Design review of the part built by this model. Coordinates are the model's own, in mm. A direction names the side the tool comes from. Coordinates: 2 decimals unless noted, no trailing zeros. Write each loop counter-clockwise with the first axis right and the second up, starting at its lowest first coordinate (ties: lowest second). Pieces come first, ordered by that corner, then holes. Notation, with made-up numbers: (40, 83) -> (85, 83) arc R22 cw to (85, 118) -> close; hole circle Ø7 at (2.5, 83.25). An arc over 180 degrees is marked (long way). Answer in a Markdown table with one row per item. Add a question column.
Item 1: Take a section at D-D, the plane x = 65. Write out the cut boundary in (y, z).
Item 2: To check wall thickness, follow line 1 (Z direction, x = -124, y = 12.75); line 2 (Z direction, x = -187, y = 11); line 3 (X direction, y = 25.75, z = 16). State the ranges of each line that lie inside material, in increasing order.
Item 3: Clearance check with flat-ended pins moving along their axes: P1, Ø9, axis at x = -237, z = 0, coming from the +Y side; P2, Ø6, axis at x = -19, z = -0.5, coming from the -Y side; P3, Ø6, axis at x = -152, y = 12.5, coming from the -Z side; P4, Ø4, axis at y = 5.5, z = 5, coming from the +X side. State where each tip first meets the part, or that it passes through.
Item 4: Take a section at C-C, the plane z = 29. Write out the cut boundary in (x, y).
Item 5: Take a section at A-A, the plane x = -77. Write out the cut boundary in (y, z), and give its area (3 significant figures).
Item 6: For faces 1 (the face through (80.096, 20.14, -5.42)), 2 (the face through (-234, 21, 0)), 3 (the face through (-98, 15, -17.5)), list the 3-axis set-ups (+Z, -Z, +X, -X, +Y, -Y) from which the entire face can be reached by the end or side of a thin tool; tool diameter is ignored.
Item 7: Draft analysis for pull direction X (two halves, no side actions). For faces 4 (the face through (144.484, 15.21, 1.174)), 5 (the face through (-124, 15, -9.538)), 6 (the face through (-98, 15, 17.5)), state which applies: released by +X, released by -X, zero draft, split by the parting line, or undercut.
Item 8: Take a section at B-B, the plane y = 26.5. Write out the cut boundary in (x, z).
from build123d import *

# Parameters (mm, degrees)
SKETCH2_W           = 247
SKETCH2_H           = 35
BOSS_EXTRUDE1_DEPTH = 30
SKETCH3_R           = 5.6
CUT_EXTRUDE1_DEPTH  = 250.429849858
CUT_EXTRUDE2_DEPTH  = 22
SKETCH6_W           = 22.496439662
SKETCH6_H           = 14
BOSS_EXTRUDE3_DEPTH = 38
CUT_EXTRUDE4_DEPTH  = 17.5
SKETCH9_R           = 2
CUT_EXTRUDE5_DEPTH  = 38
SKETCH15_R          = 2.75
CUT_EXTRUDE10_DEPTH = 9
CUT_EXTRUDE11_DEPTH = 21
SKETCH17_W          = 129.66543269
SKETCH17_H          = 19.076880406
CUT_EXTRUDE12_DEPTH = 250.429849858
FILLET1_R           = 10
SKETCH19_W          = 35
SKETCH19_H          = 30
BOSS_EXTRUDE5_DEPTH = 55
BOSS_EXTRUDE4_DEPTH = 30
SKETCH21_R          = 25
CUT_EXTRUDE14_DEPTH = 20


with BuildPart() as part:
    # Sketch2 → Boss-Extrude1 (new body)
    with BuildSketch(Plane(origin=(0, 0, 0), x_dir=(1, 0, 0), z_dir=(0, 1, 0))):
        with Locations((-123.5, 0)):
            Rectangle(SKETCH2_W, SKETCH2_H)
    extrude(amount=BOSS_EXTRUDE1_DEPTH)

    # Sketch3 → Cut-Extrude1 (cut, through all)
    with BuildSketch(Plane.XZ):
        with Locations(Location((-21, 0, 0), (0, 0, 270))):
            Circle(SKETCH3_R)
    extrude(amount=-CUT_EXTRUDE1_DEPTH, mode=Mode.SUBTRACT)

    # Sketch4 → Cut-Extrude2 (cut)
    with BuildSketch(Plane(origin=(0, 30, 0), x_dir=(1, 0, 0), z_dir=(0, 1, 0))):
        Polygon((-14.9, 3.521836642), (-21, 7.043673284), (-27.1, 3.521836642), (-27.1, -3.521836642), (-21, -7.043673284), (-14.9, -3.521836642), align=None)
    extrude(amount=-CUT_EXTRUDE2_DEPTH, mode=Mode.SUBTRACT)

    # Sketch6 → Boss-Extrude3 (add)
    with BuildSketch(Plane(origin=(0, 0, 0), x_dir=(0, 0, -1), z_dir=(1, 0, 0))):
        with Locations((0.204742288, 23)):
            Rectangle(SKETCH6_W, SKETCH6_H)
    extrude(amount=-BOSS_EXTRUDE3_DEPTH)

    # Sketch7 → Cut-Extrude4 (cut)
    with BuildSketch(Plane.XY.offset(17.5)):
        Polygon((-21, 16), (-14.9, 16), (-14.9, 8), (-15.4, 8), (-15.4, 0), (-26.6, 0), (-26.6, 8), (-27.1, 8), (-27.1, 16), align=None)
    extrude(amount=-CUT_EXTRUDE4_DEPTH, mode=Mode.SUBTRACT)

    # Sketch9 → Cut-Extrude5 (cut)
    with BuildSketch(Plane(origin=(0, 30, 0), x_dir=(1, 0, 0), z_dir=(0, 1, 0))):
        with Locations(Location((-21, 0, 0), (0, 0, 270))):
            Circle(SKETCH9_R)
    extrude(amount=-CUT_EXTRUDE5_DEPTH, mode=Mode.SUBTRACT)

    # Sketch15 → Cut-Extrude10 (cut)
    with BuildSketch(Plane(origin=(0, 30, 0), x_dir=(1, 0, 0), z_dir=(0, 1, 0))):
        with Locations(Location((-237, 0, 0), (0, 0, 270))):
            Circle(SKETCH15_R)
    extrude(amount=-CUT_EXTRUDE10_DEPTH, mode=Mode.SUBTRACT)

    # Sketch16 → Cut-Extrude11 (cut)
    with BuildSketch(Plane.XZ):
        Polygon((-241.130206964, 2.650419546), (-241.36043414, -2.25165438), (-237.230227176, -4.902073926), (-232.869793036, -2.650419546), (-232.63956586, 2.25165438), (-236.769772824, 4.902073926), align=None)
    extrude(amount=-CUT_EXTRUDE11_DEPTH, mode=Mode.SUBTRACT)

    # Sketch17 → Cut-Extrude12 (cut, through all)
    with BuildSketch(Plane(origin=(0, 30, 0), x_dir=(1, 0, 0), z_dir=(0, 1, 0))):
        with Locations((-123.5, 0)):
            Rectangle(SKETCH17_W, SKETCH17_H)
    extrude(amount=-CUT_EXTRUDE12_DEPTH, mode=Mode.SUBTRACT)

    # Fillet1
    # the kernel refuses this fillet: 10 mm, written as the material it adds along each edge
    with BuildSketch(Plane(origin=(-58.667283655, 30, 9.538440203), x_dir=(0, 0, -1), z_dir=(0, -1, 0))) as fillet1_piece_1:
        with BuildLine():
            CenterArc((FILLET1_R, -FILLET1_R), FILLET1_R, 90, 90)
            Line((0, -FILLET1_R), (0, 0))
            Line((0, 0), (FILLET1_R, 0))
        make_face()
    extrude(amount=30)
    with BuildSketch(Plane(origin=(-58.667283655, 30, -9.538440203), x_dir=(0, 0, 1), z_dir=(0, -1, 0)), Plane(origin=(-188.332716345, 30, -9.538440203), x_dir=(1, 0, 0), z_dir=(0, -1, 0)), Plane(origin=(-188.332716345, 30, 9.538440203), x_dir=(0, 0, -1), z_dir=(0, -1, 0))) as fillet1_piece_2:
        with BuildLine():
            CenterArc((FILLET1_R, FILLET1_R), FILLET1_R, 180, 90)
            Line((0, FILLET1_R), (0, 0))
            Line((0, 0), (FILLET1_R, 0))
        make_face()
    extrude(amount=30)

    # Sketch19 → Boss-Extrude5 (add)
    with BuildSketch(Plane(origin=(0, 0, 0), x_dir=(0, 0, -1), z_dir=(1, 0, 0))):
        with Locations((0, 15)):
            Rectangle(SKETCH19_W, SKETCH19_H)
    extrude(amount=BOSS_EXTRUDE5_DEPTH)

    # Sketch18 → Boss-Extrude4 (add)
    with BuildSketch(Plane(origin=(0, 30, 0), x_dir=(1, 0, 0), z_dir=(0, 1, 0))):
        with BuildLine():
            Line((55, 17.5), (55, -17.5))
            Line((55, -17.5), (84.405509337, -34.58567742))
            ThreePointArc((84.405509337, -34.58567742), (144.501054052, 0), (84.405509337, 34.58567742))
            Line((84.405509337, 34.58567742), (55, 17.5))
        make_face()
    extrude(amount=-BOSS_EXTRUDE4_DEPTH)

    # Sketch21 → Cut-Extrude14 (cut)
    with BuildSketch(Plane(origin=(0, 30, 0), x_dir=(1, 0, 0), z_dir=(0, 1, 0))):
        with Locations(Location((104.501054052, 0, 0), (0, 0, 270))):
            Circle(SKETCH21_R)
    extrude(amount=-CUT_EXTRUDE14_DEPTH, mode=Mode.SUBTRACT)


solid = part.part
Answers:
| question | item | result |
|---|---|---|
| 1 | outline | (0, -23.31) -> (30, -23.31) -> (30, 23.31) -> (0, 23.31) -> close |
| 2 | line 1 | z = -17.5 to -9.54, 9.54 to 17.5 |
| 2 | line 2 | z = -17.5 to -4.53, 4.53 to 17.5 |
| 2 | line 3 | x = -247 to 85.29, 123.71 to 141.16 |
| 3 | P1 | stops at y = 30 |
| 3 | P2 | stops at y = 16 |
| 3 | P3 | stops at z = -17.5 |
| 3 | P4 | stops at x = 144.39 |
| 4 | outline | (74.79, 0) -> (132.05, 0) -> (132.05, 30) -> (74.79, 30) -> close |
| 5 | outline | (0, -17.5) -> (30, -17.5) -> (30, -9.54) -> (0, -9.54) -> close; (0, 9.54) -> (30, 9.54) -> (30, 17.5) -> (0, 17.5) -> close |
| 5 | area | 478 mm^2 |
| 6 | face 1 | +Y |
| 6 | face 2 | -Y |
| 6 | face 3 | -Z, -X, +Y, -Y |
| 7 | face 4 | split by the parting line |
| 7 | face 5 | undercut |
| 7 | face 6 | zero draft |
| 8 | outline | (-247, -17.5) -> (55, -17.5) -> (84.41, -34.59) arc R40 ccw (long way) to (84.41, 34.59) -> (55, 17.5) -> (-247, 17.5) -> close; hole circle Ø5.5 at (-237, 0); hole (-188.32, 0) arc R10 ccw to (-178.33, -9.54) -> (-68.67, -9.54) arc R10 ccw to (-58.68, 0) arc R10 ccw to (-68.67, 9.54) -> (-178.33, 9.54) arc R10 ccw to start; hole circle Ø4 at (-21, 0); hole circle Ø50 at (104.5, 0) |
